Here's how the part is built. I have some questions about the finished solid (model axes, mm). A direction names the side the tool comes from. Round coordinates to 2 decimals unless told otherwise and drop trailing zeros. Loops run counter-clockwise (first coordinate to the right, second up) from the corner with the lowest first, then second, coordinate; pieces in that order, holes last. Notation, with made-up numbers: M -35,61 L 20,61 A20 cw 20,73 Z; hole C -34.5,80 d11. An arc over 180 degrees is marked long. Use a Markdown table: item, result.
```python
from build123d import *

# Parameters (mm, degrees)
SKETCH1_R           = 12.6365
BOSS_EXTRUDE1_DEPTH = 79.375
SKETCH2_R           = 12.7
BOSS_EXTRUDE2_DEPTH = 82.55
SKETCH3_R           = 12.6365
BOSS_EXTRUDE3_DEPTH = 79.375
CHAMFER1_SIZE       = 3.175
CUT_EXTRUDE1_DEPTH  = 57.15
CUT_EXTRUDE2_START  = -241.3
CUT_EXTRUDE2_DEPTH  = 57.15
CUT_EXTRUDE3_START  = -120.65
CUT_EXTRUDE3_DEPTH  = 19.05


with BuildPart() as part:
    # Sketch1 → Boss-Extrude1 (new body)
    with BuildSketch(Plane(origin=(0, 0, 0), x_dir=(0, 0, -1), z_dir=(1, 0, 0))):
        Circle(SKETCH1_R)
    extrude(amount=-BOSS_EXTRUDE1_DEPTH)

    # Sketch2 → Boss-Extrude2 (add)
    with BuildSketch(Plane.ZY.offset(79.375)):
        Circle(SKETCH2_R)
    extrude(amount=BOSS_EXTRUDE2_DEPTH)

    # Sketch3 → Boss-Extrude3 (add)
    with BuildSketch(Plane.ZY.offset(161.925)):
        Circle(SKETCH3_R)
    extrude(amount=BOSS_EXTRUDE3_DEPTH)

    # Chamfer1
    chamfer1_edges = [part.edges().sort_by_distance(p)[0] for p in [
        (-241.3, 0, -12.6365),
        (0, 0, 12.6365),
    ]]
    chamfer(chamfer1_edges, length=CHAMFER1_SIZE)

    # Sketch4 → Cut-Extrude1 (cut)
    with BuildSketch(Plane(origin=(0, 0, 0), x_dir=(0, 0, -1), z_dir=(1, 0, 0))):
        with BuildLine():
            Line((-2.3876, 11.176), (2.3876, 11.176))
            Line((2.3876, 11.176), (2.3876, 12.473546658))
            ThreePointArc((2.3876, 12.473546658), (0, 12.7), (-2.3876, 12.473546658))
            Line((-2.3876, 12.473546658), (-2.3876, 11.176))
        make_face()
    extrude(amount=-CUT_EXTRUDE1_DEPTH, mode=Mode.SUBTRACT)

    # Sketch4<2> → Cut-Extrude2 (cut)
    with BuildSketch(Plane(origin=(0, 0, 0), x_dir=(0, 0, -1), z_dir=(1, 0, 0)).offset(CUT_EXTRUDE2_START)):
        with BuildLine():
            Line((-2.3876, 11.176), (2.3876, 11.176))
            Line((2.3876, 11.176), (2.3876, 12.473546658))
            ThreePointArc((2.3876, 12.473546658), (0, 12.7), (-2.3876, 12.473546658))
            Line((-2.3876, 12.473546658), (-2.3876, 11.176))
        make_face()
    extrude(amount=CUT_EXTRUDE2_DEPTH, mode=Mode.SUBTRACT)

    # Sketch4<4> → Cut-Extrude3 (cut, symmetric)
    with BuildSketch(Plane(origin=(0, 0, 0), x_dir=(0, 0, -1), z_dir=(1, 0, 0)).offset(CUT_EXTRUDE3_START)):
        with BuildLine():
            Line((-2.3876, 11.176), (2.3876, 11.176))
            Line((2.3876, 11.176), (2.3876, 12.473546658))
            ThreePointArc((2.3876, 12.473546658), (0, 12.7), (-2.3876, 12.473546658))
            Line((-2.3876, 12.473546658), (-2.3876, 11.176))
        make_face()
    extrude(amount=CUT_EXTRUDE3_DEPTH, both=True, mode=Mode.SUBTRACT)


solid = part.part
```
Q1. Will these pins go through, and if not, where does the flat tip stop? P1, Ø0.7, axis at y = 12, z = -0.5, coming from the -X side; P2, Ø6, axis at x = -87.5, y = 8.5, coming from the +Z side; P3, Ø1.4, axis at x = -216, z = -1, coming from the +Y side.
Return value:
| item | result |
|---|---|
| P1 | stops at x = -184.15 |
| P2 | stops at z = 11.45 |
| P3 | stops at y = 11.18 |
Q2. We'd pull the mould along Z, two halves only. Please class faces 1 (the flat face through (-241.3, 0, 0)), 2 (the cylindrical face through (-120.07, -12.4, -2.75)), 3 (the flat face through (-212, 11.176, 0)): pulls with the +Z half, pulls with the -Z half, needs draft (parallel to the pull), parting line crosses it, or undercut.
Return value:
| item | result |
|---|---|
| face 1 | needs draft |
| face 2 | parting line crosses it |
| face 3 | undercut |
Q3. I need wall thicknesses on line 1 (Y direction, x = -159, z = -1.25); line 2 (Y direction, x = -120, z = -8.5); line 3 (Z direction, x = -84.5, y = -1). Which ranges of each line are inside material? Lowest first, please. Write a range as from..to.
Return value:
| item | result |
|---|---|
| line 1 | y = -12.64..12.64 |
| line 2 | y = -9.44..9.44 |
| line 3 | z = -12.66..12.66 |
Q4. For faces 4 (the flat face through (-120, 11.176, 0)), 5 (the flat face through (-29, 11.176, 0)), which set-ups out of +Z, -Z, +X, -X, +Y, -Y let a thin tool reach every point of the face, with its end or its side?
Return value:
| item | result |
|---|---|
| face 4 | +Y |
| face 5 | +X, +Y |
Q5. Imagine slicing it at B-B, the plane x = -16. Please give me the cut outline in (y, z), then the cut area to 3 significant figures.
Return value:
| item | result |
|---|---|
| outline | M 11.18,-2.39 L 11.18,2.39 L 12.41,2.39 A12.64 ccw long 12.41,-2.39 Z |
| area | 495 mm^2 |
